Autodesk Inventor part; units mm, degrees
ref_plane "작업 평면3" through (0, 0, 27) normal (0, 0, 1) x (1, 0, 0)
ref_plane "작업 평면4" through (-50, 28.8532, 6.8404) normal (0, -0.9397, 0.342) x (1, 0, 0)
ref_plane "YZ Plane" through (0, 0, 0) normal (1, 0, 0) x (0, 1, 0)
sketch "스케치2" plane through (0, 0, 0) normal (1, 0, 0) x (0, 1, 0)
  line L0 (-42.3529, 0) -> (47.6471, 0) construction
  line L1 (47.6471, 0) -> (-27.5284, 27.3616)
  line L2 (-27.5284, 27.3616) -> (-42.3529, 0)
  line L3 (47.6471, 0) -> (-42.3529, 0) construction
  line L4 (-42.3529, 0) -> (-42.3529, -4)
  line L5 (-42.3529, -4) -> (47.6471, -4)
  line L6 (47.6471, -4) -> (47.6471, 0)
  point P0 (0, 0)
  dimension "d2" = 90
  dimension "d3" = 80
  dimension "d4" = 20
  dimension "d7" = 4
extrude "돌출2" add sketch "스케치2" along normal mid plane 80
sketch "스케치3" plane through (40, 47.6471, -4) normal (0, 0, -1) x (-1, 0, 0)
  line L0 (80, 0) -> (0, 0)
  line L1 (0, -10) -> (40, -10)
  line L2 (80, -90) -> (0, -90)
  line L3 (0, -75.1754) -> (0, -90)
  line L4 (0, -80) -> (80, -80)
  line L5 (80, 0) -> (80, -90)
  line L6 (40, -93) -> (40, 7) construction
  circle A0 centre (40, -80) radius 2.5
  circle A1 centre (40, -10) radius 2.5
  line L7 (0, 0) -> (0, -75.1754)
  point P0 (40, -47.6471)
  dimension "d10" = 10
  dimension "d12" = 10
  dimension "d13" = 5
  dimension "d14" = 5
  dimension "d44" = 40
extrude "돌출3" cut sketch "스케치3" against normal blind 40 contours A1 | A0 L4 | L4 A0
ref_plane "작업 평면3" through (0, 0, 27) normal (0, 0, 1) x (1, 0, 0)
sketch "스케치4" plane through (0, 0, 27) normal (0, 0, 1) x (1, 0, 0)
  circle A0 centre (0, 37.6471) radius 2.5
  circle A1 centre (0, -32.3529) radius 2.5
  circle A2 centre (0, 37.6471) radius 3.5
  circle A3 centre (0, -32.3529) radius 3.5
  point P0 (0, 0)
  dimension "d18" = 7
  dimension "d19" = 7
extrude "돌출4" cut sketch "스케치4" against normal blind 27 contours A0 | A1 | A2 | A3
sketch "스케치5" plane through (-40, -27.5284, 27.3616) normal (0, 0.342, 0.9397) x (1, 0, 0)
  line L0 (20, 80) -> (20, -25) construction
  line L1 (-10, 60) -> (63, 60) construction
  line L2 (0, 80) -> (80, 80)
  point P0 (40, 35.2264)
  dimension "d22" = 20
ref_plane "작업 평면4" through (-50, 28.8532, 6.8404) normal (0, -0.9397, 0.342) x (1, 0, 0)
sketch "스케치6" plane through (-50, 28.8532, 6.8404) normal (0, -0.9397, 0.342) x (1, 0, 0)
  line L0 (50, 15) -> (50, -51) construction
  line L1 (46.5, 0) -> (53.5, 0)
  line L2 (10, 0) -> (90, 0)
  line L3 (21, 0) -> (21, 0)
  line L4 (90, 0) -> (90, -30.7818)
  line L5 (39.1, 0) -> (41, 0)
  line L6 (41, 0) -> (41, 2)
  line L7 (39.1, 2) -> (39.1, 0)
  line L8 (36.05, 3.5) -> (44.05, 3.5)
  line L9 (44.05, 3.5) -> (44.05, 2)
  line L10 (36.05, 2) -> (36.05, 3.5)
  line L11 (44.05, 2) -> (41, 2)
  line L12 (39.1, 2) -> (36.05, 2)
  line L13 (59, 0) -> (59, 2)
  line L14 (60.9, 2) -> (60.9, 0)
  line L15 (63.95, 3.5) -> (55.95, 3.5)
  line L16 (55.95, 3.5) -> (55.95, 2)
  line L17 (63.95, 2) -> (63.95, 3.5)
  line L18 (55.95, 2) -> (59, 2)
  line L19 (60.9, 2) -> (63.95, 2)
  line L20 (10, -30.7818) -> (10, 0)
  point P0 (50, -16.2963)
  point P1 (41, 1)
  point P2 (59, 1)
  point P3 (59, 0)
  point P4 (60.9, 0)
  dimension "d30" = 9
  dimension "d35" = 8
  dimension "d36" = 1.5
  dimension "d37" = 2
  dimension "d38" = 3.05
  dimension "d41" = 1.5
  dimension "d42" = 3.05
  dimension "d43" = 40
extrude "돌출5" add sketch "스케치6" along normal mid plane 12
properties part number "LCD_Mount_20degrees"
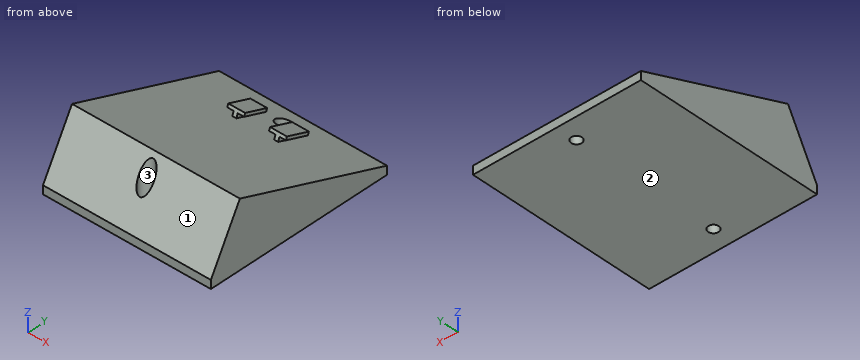
For this review, take the finished solid that the model builds, in its own axes (mm). Face numbers are marked on the shaded views. Give positions to 0.01 mm unless a question says otherwise; leave off trailing zeros. Write each loop counter-clockwise with the first axis right and the second up, starting at its lowest first coordinate (ties: lowest second). Pieces come first, ordered by that corner, then holes.
Item 1: Take a section at A-A (x = -12). Give the boundary of the cut face in (y, z).
Item 2: Take a section at D-D (z = 22.5). Give the boundary of the cut face in (x, y).
Item 3: Take a section at B-B (x = 0). Give the boundary of the cut face in (y, z), and give its area (3 significant figures).
Item 4: Insertion check: P1, Ø5.5, axis at x = 0, y = 37.65, coming from the +Z side; P2, Ø1.5, axis at x = 8, z = 1.5, coming from the -Y side; P3, Ø1, axis at x = 14.5, y = -31, coming from the +Z side. Each pin has a flat end and moves straight along its axis. Give the tip position at first contact, or say it passes through.
Item 5: The part is to be moulded in two halves that separate along Y. For the marked faces 1, 2 and 3, say which applies: +Y half, -Y half, draft (parallel to the pull), parting line (faces both ways), or undercut.
Item 6: Wall thickness on probe 1 along Y at (x, z) = (0, -1); probe 2 along Z at (x, y) = (-1.5, -2); probe 3 along Z at (x, y) = (-4, 41.5): over which ranges is each line inside the solid? List them lowest first.
Item 7: Take a section at C-C (x = -26.5). Give the boundary of the cut face in (y, z).
Established:
1. outline: (-42.35, -4) - (47.65, -4) - (47.65, 0) - (-27.53, 27.36) - (-42.35, 0) - close; (23.9, 10.77) - (35.18, 6.67) - (35.69, 8.08) - (24.41, 12.18) - close
2. outline: (-40, -30.16) - (-2.73, -30.16) arc R3.5 cw to (2.73, -30.16) - (40, -30.16) - (40, -14.17) - (-40, -14.17) - close
3. outline: (-42.35, -4) - (-34.85, -4) - (-34.85, 0) - (-35.85, 0) - (-35.85, 12) - (-42.35, 0) - close; (-29.85, -4) - (35.15, -4) - (35.15, 0) - (34.15, 0) - (34.15, 4.91) - (-27.53, 27.36) - (-28.85, 24.92) - (-28.85, 0) - (-29.85, 0) - close; (40.15, -4) - (47.65, -4) - (47.65, 0) - (41.15, 2.37) - (41.15, 0) - (40.15, 0) - close
3. area: 1,400 mm2
4. P1: stops at z = 0
4. P2: stops at y = -41.95
4. P3: stops at z = 21.88
5. face 1: -Y half
5. face 2: draft
5. face 3: undercut
6. probe 1: y = -42.35 to -34.85, -29.85 to 35.15, 40.15 to 47.65
6. probe 2: z = -4 to 18.07
6. probe 3: z = -4 to 2.24
7. outline: (-42.35, -4) - (47.65, -4) - (47.65, 0) - (-27.53, 27.36) - (-42.35, 0) - close
